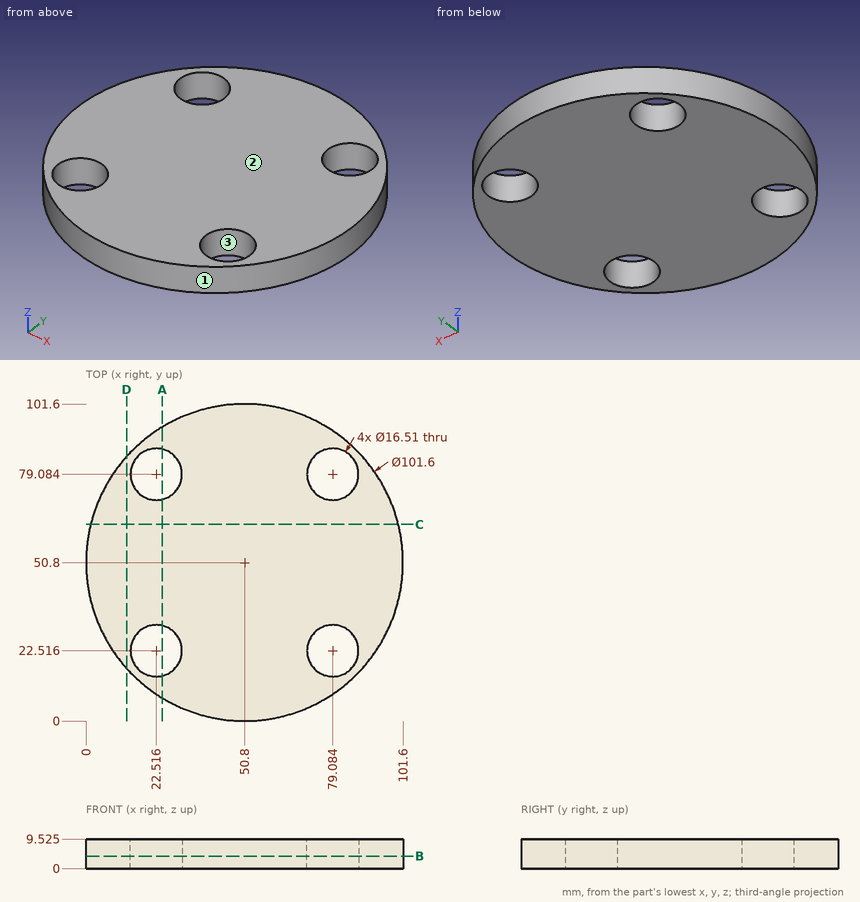
Drawing for the job (mm, zero at the part's lowest x, y, z). Coordinates: 2 decimals unless noted, no trailing zeros. Order: outer loops, then holes, each group sorted by start corner. A loop starts at its lowest first (then second) coordinate and runs counter-clockwise, first axis right, second up.
Item 1: Band-saw the part on A-A on x = 24.5. List the corners of the cut face in (y, z) (1 decimal), plus the area to 3 significant figures.
Check sheet entries:
outline: (7.3, 0) - (14.5, 0) - (14.5, 9.5) - (7.3, 9.5) - close; (30.5, 0) - (71.1, 0) - (71.1, 9.5) - (30.5, 9.5) - close; (87.1, 0) - (94.3, 0) - (94.3, 9.5) - (87.1, 9.5) - close
area: 523 mm2
Item 2: Pin check, flat tips, straight feed: pin 1 Ø1.5 at (x, z) = (10, 4) entering from -Y; pin 2 Ø1 at (y, z) = (13.5, 8) entering from -X; pin 3 Ø2 at (y, z) = (43, 3) entering from +X. Stop position of each tip, or through.
Check sheet entries:
pin 1: stops at y = 19.55
pin 2: stops at x = 15.78
pin 3: stops at x = 101.14
Item 3: Band-saw the part on D-D on x = 13. List the corners of the cut face in (y, z) (1 decimal).
Check sheet entries:
outline: (16.9, 0) - (84.7, 0) - (84.7, 9.5) - (16.9, 9.5) - close
Item 4: Two-plate mould, pull along X, no slides. Class the marked faces 1, 2 and 3: +X half, -X half, draft (parallel to the pull), parting line (faces both ways), or undercut.
Check sheet entries:
face 1: parting line
face 2: draft
face 3: undercut
Item 5: Drill centre lines: L1, parallel to Y at x = 20, z = 6.5; L2, parallel to Y at x = 77.5, z = 5.5 (1 decimal); L3, parallel to X at y = 16, z = 8 (1 decimal). Where is each one in solid material? Low to high.
Check sheet entries:
L1: y = 10.4 to 14.65, 30.38 to 71.22, 86.95 to 91.2
L2: y = 7.6 to 14.4, 30.6 to 71, 87.2 to 94
L3: x = 13.8 to 17.4, 27.6 to 74, 84.2 to 87.8
Item 6: Band-saw the part on B-B on z = 4. List the corners of the cut face in (x, y) (1 decimal).
Check sheet entries:
outline: circle Ø101.6 at (50.8, 50.8); hole circle Ø16.5 at (22.5, 22.5); hole circle Ø16.5 at (22.5, 79.1); hole circle Ø16.5 at (79.1, 22.5); hole circle Ø16.5 at (79.1, 79.1)
Item 7: Band-saw the part on C-C on y = 63. List the corners of the cut face in (x, z) (1 decimal).
Check sheet entries:
outline: (1.5, 0) - (100.1, 0) - (100.1, 9.5) - (1.5, 9.5) - close
